Read the model definition and answer for the solid it produces. Units are mm, in the model's axes. Face numbers are marked on the shaded views. A direction names the side the tool comes from. Give positions to 0.01 mm unless a question says otherwise; leave off trailing zeros. Loops run counter-clockwise (first coordinate to the right, second up) from the corner with the lowest first, then second, coordinate; pieces in that order, holes last. Notation, with made-up numbers: (18.25, 45.5) - (46.25, 45.5) arc R12 cw to (46.25, 65.5) - close; hole circle Ø11 at (13.25, 5.25). An arc over 180 degrees is marked (long way). Use a Markdown table: item, result. Add a question column.
Item 1: A cutting plane is placed at C-C (x = 59.5). Determine the outline of the cut face in (y, z), plus the area to 3 significant figures.
Item 2: Each of these flat-tipped pins is pushed along its axis until it touches: P1, Ø12, axis at x = 73, z = 13, coming from the -Y side; P2, Ø1.8, axis at y = 20.5, z = 1.5, coming from the -X side; P3, Ø12, axis at x = 20.5, y = 32.5, coming from the +Z side; P4, Ø4.5, axis at y = 12.8, z = 17.35, coming from the -X side. Where does it stop, or does it pass through?
Item 3: Which of the six approach directions +Z, -Z, +X, -X, +Y, -Y give full straight-line access (tool end or side, diameter ignored) to the marked faces 1, 2, 3, 4 and 5?
Item 4: For a pull along Y with two mould halves and no side action, classify the marked faces 6, 7 and 8 as +Y half, -Y half, draft (parallel to the pull), parting line (faces both ways), or undercut.
Item 5: A cutting plane is placed at B-B (x = 77.5). Determine the outline of the cut face in (y, z), plus the area to 3 significant figures.
Item 6: A cutting plane is placed at D-D (z = 7.25). Give the number of separate pieces and of enclosed holes in the cut face, plus the area to 3 significant figures.
Item 7: A cutting plane is placed at A-A (y = 20). Determine the outline of the cut face in (x, z).
Item 8: Consider probe 1 along Z at (x, y) = (88.4, 27.3); probe 2 along Y at (x, z) = (82.5, 10.15); probe 3 along Z at (x, y) = (88, 12). Determine where each line is inside the solid, lowest interval first. Write a range as [from, to].
from build123d import *

# Parameters (mm, degrees)
BODY_DEPTH          = 10
PCB_RECESS_DEPTH    = 7.75
SKETCH11_R          = 3.000000000000004
SKETCH11_R_2        = 3.0000000000000084
SKETCH11_R_3        = 3.000000000000008
SKETCH11_R_4        = 2.999999999999999
PCB_BOSS_DEPTH      = 6.75
FILLET2_R           = 2.25
BOSS_EXTRUDE2_DEPTH = 15.25
SKETCH24_W          = 15.25
SKETCH24_H          = 9.74999999999999
SKETCH24_W_2        = 15.249999999999972
SKETCH24_H_2        = 9.750000000000002
BOSS_EXTRUDE3_DEPTH = 3
SKETCH25_R          = 6.5
CUT_EXTRUDE9_DEPTH  = 15
CUT_EXTRUDE10_DEPTH = 2.25
FILLET7_R           = 3
FILLET8_R           = 2.25
SKETCH27_R          = 2.0000000000000067
SKETCH27_R_2        = 2.000000000000003
SKETCH27_R_3        = 2
SKETCH27_R_4        = 1.9999999999999996
CUT_EXTRUDE11_DEPTH = 5.5
BOSS_EXTRUDE4_DEPTH = 6.75
SKETCH12_R          = 1.9999999999999991
SKETCH12_R_2        = 1.9999999999999967
SKETCH12_R_3        = 1.9999999999999996
CUT_EXTRUDE5_DEPTH  = 4.5


with BuildPart() as part:
    # Sketch4 → body (new body)
    with BuildSketch(Plane.XY):
        Polygon((0, 40), (1.73e-15, 25.25), (14.7, 25.25), (14.7, 14.750000000000002), (0, 14.75), (0, 0), (89.99999999999999, -6.94e-15), (90, 39.99999999999999), align=None)
    extrude(amount=BODY_DEPTH)

    # Sketch10 → pcb-recess (cut)
    with BuildSketch(Plane.XY.offset(10)):
        Polygon((72.75000000000001, 2.250000000000009), (2.2500000000000018, 2.2500000000000004), (2.2500000000000044, 37.74999999999999), (72.75, 37.75000000000001), align=None)
    extrude(amount=-PCB_RECESS_DEPTH, mode=Mode.SUBTRACT)

    # Sketch11 → pcb-boss (add)
    with BuildSketch(Plane.XY.offset(2.25)):
        with Locations((6.000000000000004, 34)):
            Circle(SKETCH11_R)
        with Locations((69, 34)):
            Circle(SKETCH11_R_2)
        with Locations((69, 6.000000000000005)):
            Circle(SKETCH11_R_3)
        with Locations((6.000000000000007, 6.000000000000005)):
            Circle(SKETCH11_R_4)
    extrude(amount=PCB_BOSS_DEPTH)

    # Fillet2
    fillet2_edges = [part.edges().sort_by_distance(p)[0] for p in [
        (0, 14.75, 5),
        (1.73e-15, 25.25, 5),
    ]]
    fillet(fillet2_edges, radius=FILLET2_R - 0.0001)  # a hair under: the kernel refuses the full size

    # Sketch23 → Boss-Extrude2 (add)
    with BuildSketch(Plane(origin=(89.99999999999999, -3.123e-14, 0), x_dir=(0, 0, -1), z_dir=(1, -3.5e-16, 0))):
        Polygon((-10, 30.250000000000025), (-20.299999999999997, 30.25000000000003), (-20.299999999999994, 9.750000000000027), (-9.999999999999998, 9.75000000000002), align=None)
    extrude(amount=-BOSS_EXTRUDE2_DEPTH)

    # Sketch24 → Boss-Extrude3 (add)
    with BuildSketch(Plane.XY.offset(10)):
        with Locations((82.375, 35.125)):
            Rectangle(SKETCH24_W, SKETCH24_H)
        with Locations((82.375, 4.874999999999994)):
            Rectangle(SKETCH24_W_2, SKETCH24_H_2)
    extrude(amount=BOSS_EXTRUDE3_DEPTH)

    # Sketch25 → Cut-Extrude9 (cut)
    with BuildSketch(Plane(origin=(89.99999999999999, -3.123e-14, 0), x_dir=(0, 0, -1), z_dir=(1, -3.5e-16, 0))):
        with Locations(Location((-10.149999999999999, 20.000000000000025, 0), (0, 0, 90))):
            Circle(SKETCH25_R)
    extrude(amount=-CUT_EXTRUDE9_DEPTH, mode=Mode.SUBTRACT)

    # Sketch26 → Cut-Extrude10 (cut)
    with BuildSketch(Plane(origin=(75, -2.602e-14, 0), x_dir=(0, 0, -1), z_dir=(1, -3.5e-16, 0))):
        with BuildLine():
            Line((-10.149999999999999, 26.500000000000025), (-10.149999999999999, 13.500000000000027))
            ThreePointArc((-10.149999999999999, 13.500000000000027), (-3.6499999999999986, 20.000000000000025), (-10.149999999999999, 26.500000000000025))
        make_face()
    extrude(amount=-CUT_EXTRUDE10_DEPTH, mode=Mode.SUBTRACT)

    # Fillet7
    fillet7_edges = [part.edges().sort_by_distance(p)[0] for p in [
        (82.375, 9.749999999999995, 13),
        (82.37499999999999, 9.749999999999996, 20.299999999999994),
        (82.375, 30.25, 20.299999999999997),
        (82.375, 30.25, 13),
    ]]
    fillet(fillet7_edges, radius=FILLET7_R)

    # Fillet8
    fillet8_edges = [part.edges().sort_by_distance(p)[0] for p in [
        (0, 40, 5),
        (90, 39.99999999999999, 6.5),
        (89.99999999999999, -6.94e-15, 6.5),
        (0, 0, 5),
    ]]
    fillet(fillet8_edges, radius=FILLET8_R)

    # Sketch27 → Cut-Extrude11 (cut)
    with BuildSketch(Plane(origin=(89.99999999999999, -3.123e-14, 0), x_dir=(0, 0, -1), z_dir=(1, -3.5e-16, 0))):
        with Locations(Location((-17.350000000000005, 27.300000000000026, 0), (0, 0, 90))):
            Circle(SKETCH27_R)
        with Locations(Location((-2.850000000000002, 27.300000000000026, 0), (0, 0, 90))):
            Circle(SKETCH27_R_2)
        with Locations(Location((-2.8499999999999948, 12.800000000000026, 0), (0, 0, 90))):
            Circle(SKETCH27_R_3)
        with Locations(Location((-17.349999999999998, 12.800000000000026, 0), (0, 0, 90))):
            Circle(SKETCH27_R_4)
    extrude(amount=-CUT_EXTRUDE11_DEPTH, mode=Mode.SUBTRACT)

    # Sketch28 → Boss-Extrude4 (add)
    with BuildSketch(Plane.XY.offset(2.25)):
        with BuildLine():
            Line((6.000000000000004, 31), (2.2500000000000036, 31))
            Line((2.2500000000000036, 31), (2.2500000000000044, 37.74999999999999))
            Line((2.2500000000000044, 37.74999999999999), (9.000000000000007, 37.74999999999999))
            Line((9.000000000000007, 37.74999999999999), (9.000000000000007, 34))
            ThreePointArc((9.000000000000007, 34), (8.121320343559649, 31.878679656440355), (6.000000000000004, 31))
        make_face()
        with BuildLine():
            Line((65.99999999999999, 37.75000000000001), (65.99999999999999, 34.000000000000014))
            ThreePointArc((65.99999999999999, 34.000000000000014), (66.87867965644034, 31.878679656440372), (68.99999999999999, 31.000000000000014))
            Line((68.99999999999999, 31.000000000000014), (72.75, 31.000000000000014))
            Line((72.75, 31.000000000000014), (72.75, 37.75000000000001))
            Line((72.75, 37.75000000000001), (65.99999999999999, 37.75000000000001))
        make_face()
        with BuildLine():
            Line((68.99999999999999, 8.999999999999988), (72.75, 8.999999999999988))
            Line((72.75, 8.999999999999988), (72.75, 2.249999999999995))
            Line((72.75, 2.249999999999995), (65.99999999999999, 2.249999999999995))
            Line((65.99999999999999, 2.249999999999995), (65.99999999999999, 5.999999999999985))
            ThreePointArc((65.99999999999999, 5.999999999999985), (66.87867965644034, 8.121320343559628), (68.99999999999999, 8.999999999999988))
        make_face()
        with BuildLine():
            Line((9.000000000000007, 2.250000000000009), (9.000000000000007, 5.999999999999998))
            ThreePointArc((9.000000000000007, 5.999999999999998), (8.121320343559649, 8.121320343559642), (6.000000000000004, 9.000000000000002))
            Line((6.000000000000004, 9.000000000000002), (2.2500000000000036, 9.000000000000002))
            Line((2.2500000000000036, 9.000000000000002), (2.2500000000000044, 2.250000000000009))
            Line((2.2500000000000044, 2.250000000000009), (9.000000000000007, 2.250000000000009))
        make_face()
    extrude(amount=BOSS_EXTRUDE4_DEPTH)

    # Sketch12 → Cut-Extrude5 (cut)
    with BuildSketch(Plane.XY.offset(9.000000000000002)):
        with Locations((6.000000000000004, 34)):
            Circle(SKETCH12_R)
        with Locations((69, 34)):
            Circle(SKETCH12_R_2)
        with Locations((69, 6.000000000000005)):
            Circle(SKETCH12_R_2)
        with Locations((6.000000000000007, 6.000000000000005)):
            Circle(SKETCH12_R_3)
    extrude(amount=-CUT_EXTRUDE5_DEPTH, mode=Mode.SUBTRACT)


solid = part.part
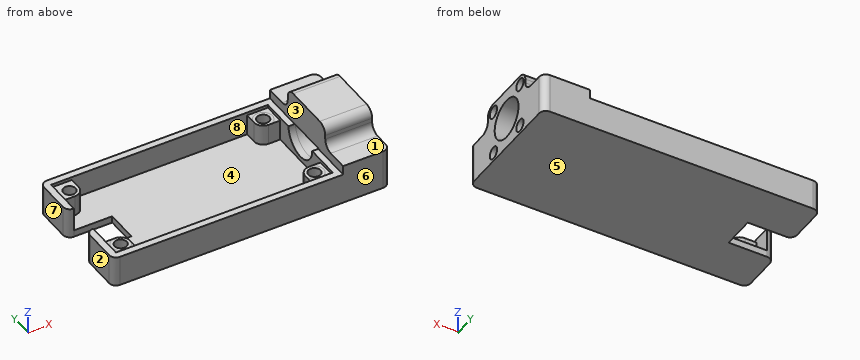
Geometry says:
| question | item | result |
|---|---|---|
| 1 | outline | (0, 0) - (40, 0) - (40, 10) - (37.75, 10) - (37.75, 2.25) - (2.25, 2.25) - (2.25, 10) - (0, 10) - close |
| 1 | area | 125 mm² |
| 2 | P1 | y = 0 |
| 2 | P2 | x = 14.7 |
| 2 | P3 | z = 10 |
| 2 | P4 | x = 74.75 |
| 3 | face 1 | +Z, +X, -X, -Y |
| 3 | face 2 | +Z, -Z, -X, +Y, -Y |
| 3 | face 3 | +Z, -X, +Y, -Y |
| 3 | face 4 | +Z |
| 3 | face 5 | -Z, +X, -X, +Y, -Y |
| 4 | face 6 | -Y half |
| 4 | face 7 | draft |
| 4 | face 8 | undercut |
| 5 | outline | (0, 0) - (40, 0) - (40, 13) - (33.25, 13) arc R3 cw to (30.25, 16) - (30.25, 17.3) arc R3 ccw to (27.25, 20.3) - (12.75, 20.3) arc R3 ccw to (9.75, 17.3) - (9.75, 16) arc R3 cw to (6.75, 13) - (0, 13) - close; hole circle Ø13 at (20, 10.15) |
| 5 | area | 537 mm² |
| 6 | separate pieces | 2 |
| 6 | enclosed holes | 4 |
| 6 | area | 991 mm² |
| 7 | outline | (14.7, 0) - (90, 0) - (90, 3.65) - (72.75, 3.65) - (72.75, 2.25) - (14.7, 2.25) - close; (74.75, 10.15) - (75, 10.15) - (75, 16.65) - (90, 16.65) - (90, 20.3) - (74.75, 20.3) - close |
| 8 | probe 1 | [0, 0.85], [4.85, 15.35], [19.35, 20.3] |
| 8 | probe 2 | [0, 13.5], [26.5, 40] |
| 8 | probe 3 | [0, 1.02], [4.68, 15.52], [19.18, 20.2] |
